```python
from build123d import *

# Parameters (mm, degrees)
SZKIC1_W                                             = 138
SZKIC1_H                                             = 60
SZKIC1_R                                             = 17
DODANIE_WYCI_GNI_CIE1_DEPTH                          = 12
POG_BIENIE_WALCOWE_POD_M5_WKR_T_DO_CZ_CI_D           = 5.5
POG_BIENIE_WALCOWE_POD_M5_WKR_T_DO_CZ_CI_CBORE_D     = 11
POG_BIENIE_WALCOWE_POD_M5_WKR_T_DO_CZ_CI_CBORE_DEPTH = 6.5
WYTNIJ_WYCI_GNI_CIE1_DEPTH                           = 5
WYTNIJ_WYCI_GNI_CIE2_DEPTH                           = 367.809214715


with BuildPart() as part:
    # Szkic1 → Dodanie-wyciągnięcie1 (new body)
    with BuildSketch(Plane.XY):
        with Locations((-1, 330)):
            Rectangle(SZKIC1_W, SZKIC1_H)
        with Locations((33.5, 330)):
            Circle(SZKIC1_R, mode=Mode.SUBTRACT)
    extrude(amount=DODANIE_WYCI_GNI_CIE1_DEPTH)

    # Pogłębienie walcowe pod M5 Wkręt do części metalowych z łbem sześciokątnym1 (through all)
    with Locations(Plane.XY.offset(12)):
        with Locations((-61, 351), (-19, 351), (-61, 309), (-19, 309)):
            CounterBoreHole(POG_BIENIE_WALCOWE_POD_M5_WKR_T_DO_CZ_CI_D / 2, POG_BIENIE_WALCOWE_POD_M5_WKR_T_DO_CZ_CI_CBORE_D / 2, POG_BIENIE_WALCOWE_POD_M5_WKR_T_DO_CZ_CI_CBORE_DEPTH)

    # Szkic5 → Wytnij-wyciągnięcie1 (cut)
    with BuildSketch(Plane(origin=(0, 0, 0), x_dir=(-1, 0, 0), z_dir=(0, 0, -1))):
        with BuildLine():
            Line((-12.93, 358.07), (-6.93, 358.07))
            ThreePointArc((-6.93, 358.07), (-2.43, 353.57), (-6.93, 349.07))
            Line((-6.93, 349.07), (-12.93, 349.07))
            ThreePointArc((-12.93, 349.07), (-17.43, 353.57), (-12.93, 358.07))
        make_face()
        with BuildLine():
            Line((-60.07, 358.07), (-54.07, 358.07))
            ThreePointArc((-54.07, 358.07), (-49.57, 353.57), (-54.07, 349.07))
            Line((-54.07, 349.07), (-60.07, 349.07))
            ThreePointArc((-60.07, 349.07), (-64.57, 353.57), (-60.07, 358.07))
        make_face()
    wytnij_wyci_gni_cie1 = extrude(amount=-WYTNIJ_WYCI_GNI_CIE1_DEPTH, mode=Mode.SUBTRACT)

    # Szkic7 → Wytnij-wyciągnięcie2 (cut, through all)
    with BuildSketch(Plane(origin=(0, 0, 5), x_dir=(-1, 0, 0), z_dir=(0, 0, -1))):
        with BuildLine():
            Line((-60.07, 350.57), (-54.07, 350.57))
            ThreePointArc((-54.07, 350.57), (-51.07, 353.57), (-54.07, 356.57))
            Line((-54.07, 356.57), (-60.07, 356.57))
            ThreePointArc((-60.07, 356.57), (-63.07, 353.57), (-60.07, 350.57))
        make_face()
        with BuildLine():
            Line((-12.93, 350.57), (-6.93, 350.57))
            ThreePointArc((-6.93, 350.57), (-3.93, 353.57), (-6.93, 356.57))
            Line((-6.93, 356.57), (-12.93, 356.57))
            ThreePointArc((-12.93, 356.57), (-15.93, 353.57), (-12.93, 350.57))
        make_face()
    wytnij_wyci_gni_cie2 = extrude(amount=-WYTNIJ_WYCI_GNI_CIE2_DEPTH, mode=Mode.SUBTRACT)

    # Lustro1: Wytnij-wyciągnięcie1, Wytnij-wyciągnięcie2 across plane
    add(wytnij_wyci_gni_cie1.mirror(Plane.ZX.offset(330)), mode=Mode.SUBTRACT)
    add(wytnij_wyci_gni_cie2.mirror(Plane.ZX.offset(330)), mode=Mode.SUBTRACT)


solid = part.part
```
Check sheet for the modelled part. Datum: model origin and axes. Units: mm. A direction names the side the tool comes from. Coordinates: 2 decimals unless noted, no trailing zeros. Order: outer loops, then holes, each group sorted by start corner. A loop starts at its lowest first (then second) coordinate and runs counter-clockwise, first axis right, second up. Notation, with made-up numbers: M -18.75,-36 L 0.25,-36 A23 ccw 0.25,-5 Z; hole C 17.5,88.25 d11. An arc over 180 degrees is marked long. One line per question, with ' | ' between items. Start each with the question number.
Item 1: Sectioned sample at B-B on z = 7.25. Count the separate pieces of the cut face and the enclosed holes in it, and give its area (3 significant figures).
Item 2: Material ranges on line 1 (Y direction, x = -19, z = 1.95); line 2 (Y direction, x = -61, z = 10.5); line 3 (X direction, y = 305, z = 2.75), recorded low to high.
Item 3: Sectioned sample at A-A on x = -19. Record the cut outline in (y, z), and give its area (4 significant figures).
Item 4: Access from +Z, -Z, +X, -X, +Y, -Y to the whole of each face (thin tool, end or side, straight path). Record for faces 4 (the cylindrical face through (49.57, 306.33, 2.46)), 5 (the flat face through (-64, 350, 5.5)), 6 (the flat face through (57, 356.57, 8)).
Item 5: Gauge pin test, flat end, axial feed: P1, Ø2.5, axis at x = 9.5, y = 355.5, coming from the -Z side. Record the tip position at first contact, or that the pin passes through.
Item 6: Mould release check, pull along Y, two halves, no side actions. Record for faces 1 (the flat face through (57, 349.07, 2)), 2 (the flat face through (68, 330, 6)), 3 (the cylindrical face through (-16.5, 304.1, 8.8)): pulls with the +Y half, pulls with the -Y half, needs draft (parallel to the pull), parting line crosses it, or undercut.
Item 7: Sectioned sample at D-D on x = 10. Record the cut outline in (y, z).
Item 8: Sectioned sample at C-C on x = 33.5. Record the cut outline in (y, z), and give its area (3 significant figures).
Answer below:
1) separate pieces: 1 | enclosed holes: 9 | area: 6,730 mm^2
2) line 1: y = 300 to 306.25, 311.75 to 348.25, 353.75 to 360 | line 2: y = 300 to 303.5, 314.5 to 345.5, 356.5 to 360 | line 3: x = -70 to 2.66, 17.2 to 49.8, 64.34 to 68
3) outline: M 300,0 L 306.25,0 L 306.25,5.5 L 303.5,5.5 L 303.5,12 L 300,12 Z; M 311.75,0 L 348.25,0 L 348.25,5.5 L 345.5,5.5 L 345.5,12 L 314.5,12 L 314.5,5.5 L 311.75,5.5 Z; M 353.75,0 L 360,0 L 360,12 L 356.5,12 L 356.5,5.5 L 353.75,5.5 Z | area: 516.5 mm^2
4) face 4: -Z | face 5: +Z | face 6: +Z, -Z
5) P1: stops at z = 5
6) face 1: undercut | face 2: needs draft | face 3: undercut
7) outline: M 300,0 L 301.93,0 L 301.93,5 L 303.43,5 L 303.43,12 L 300,12 Z; M 309.43,5 L 310.93,5 L 310.93,0 L 349.07,0 L 349.07,5 L 350.57,5 L 350.57,12 L 309.43,12 Z; M 356.57,5 L 358.07,5 L 358.07,0 L 360,0 L 360,12 L 356.57,12 Z
8) outline: M 300,0 L 313,0 L 313,12 L 300,12 Z; M 347,0 L 360,0 L 360,12 L 347,12 Z | area: 312 mm^2
